The model under review builds one solid part; all positions refer to its coordinate system, in mm. A direction names the side the tool comes from. Round coordinates to 2 decimals unless told otherwise and drop trailing zeros. Order: outer loops, then holes, each group sorted by start corner. A loop starts at its lowest first (then second) coordinate and runs counter-clockwise, first axis right, second up. Notation, with made-up numbers: M -7.75,1 L 43.25,1 A23 ccw 43.25,28 Z; hole C 72,59.5 d3. An arc over 180 degrees is marked long. Answer as CSV lines item,"result". Start each with the question number.
from build123d import *

# Parameters (mm, degrees)
SKETCH_3_W           = 10
SKETCH_3_H           = 35
SKETCH_3_W_2         = 26
SKETCH_3_H_2         = 10
SKETCH_3_W_3         = 38
SKETCH_3_W_4         = 25
EXTRUDE_1_DEPTH      = 1
EXTRUDE_2_DEPTH      = 4
EXTRUDE_2_DEPTH_BACK = 1
SKETCH_5_W           = 25
SKETCH_5_H           = 10
SKETCH_5_W_2         = 10
SKETCH_5_H_2         = 35
EXTRUDE_3_DEPTH      = 2


with BuildPart() as part:
    # 草图3 → 凸台-拉伸1 (new body)
    with BuildSketch(Plane(origin=(0, 0, 0), x_dir=(1, 0, 0), z_dir=(0, 1, 0))):
        with Locations((19, 0)):
            Rectangle(SKETCH_3_W, SKETCH_3_H)
        with Locations((1, 0)):
            Rectangle(SKETCH_3_W_2, SKETCH_3_H_2)
        Polygon((-12, -5), (-12, 5), (-12, 22.5), (-22, 22.5), (-22, 5), (-22, -5), (-22, -22.5), (-12, -22.5), align=None)
        with Locations((-41, 0)):
            Rectangle(SKETCH_3_W_3, SKETCH_3_H_2)
        with Locations((-72.5, 0)):
            Rectangle(SKETCH_3_W_4, SKETCH_3_H_2)
    extrude(amount=EXTRUDE_1_DEPTH)

    # 草图4 → 凸台-拉伸2 (add, two sides)
    with BuildSketch(Plane.XZ) as extrude_2_sk:
        Polygon((13, -18.5), (25, -18.5), (25, 18.5), (13, 18.5), (13, 6), (-11, 6), (-11, 23.5), (-23, 23.5), (-23, 6), (-86, 6), (-86, -6), (-23, -6), (-23, -23.5), (-11, -23.5), (-11, -6), (13, -6), align=None)
        Polygon((14, -17.5), (24, -17.5), (24, 17.5), (14, 17.5), (14, 5), (-12, 5), (-12, 22.5), (-22, 22.5), (-22, 5), (-85, 5), (-85, -5), (-22, -5), (-22, -22.5), (-12, -22.5), (-12, -5), (14, -5), align=None, mode=Mode.SUBTRACT)
    extrude(amount=EXTRUDE_2_DEPTH)
    extrude(extrude_2_sk.sketch, amount=-EXTRUDE_2_DEPTH_BACK)

    # 草图5 → 凸台-拉伸3 (add)
    with BuildSketch(Plane.XZ):
        Polygon((-22, 22.5), (-22, 5), (-20, 5), (-20, -5), (-22, -5), (-22, -22.5), (-12, -22.5), (-12, -5), (-14, -5), (-14, 5), (-12, 5), (-12, 22.5), align=None)
        with Locations((-72.5, 0)):
            Rectangle(SKETCH_5_W, SKETCH_5_H)
        with Locations((19, 0)):
            Rectangle(SKETCH_5_W_2, SKETCH_5_H_2)
    extrude(amount=EXTRUDE_3_DEPTH)


solid = part.part
Item 1: Consider section C-C (x = 0). State the section outline as (y, z) points.
Item 2: Tool access review of faces 1 (the flat face through (13, -2, 12)), 2 (the flat face through (19, -2, 18.5)), 3 (the flat face through (-11, -2, -15)), 4 (the flat face through (-12, -3, -14)): name each direction out of +Z, -Z, +X, -X, +Y, -Y from which nothing blocks a thin tool from reaching the whole face with its end or side.
Item 3: Consider section D-D (z = -0.5). State the section outline as (x, y) points, and give its area (3 significant figures).
Item 4: The part is to be moulded in two halves that separate along Z. For faces 5 (the flat face through (-17, -2, 23.5)), 6 (the flat face through (-11, -2, 15)), 7 (the flat face through (1, -2, -6)), 8 (the flat face through (-17, -2, 0)), say which applies: +Z half, -Z half, draft (parallel to the pull), parting line (faces both ways), or undercut.
Item 5: Consider section B-B (z = 7). State the section outline as (x, y) points, and give its area (3 significant figures).
Item 6: For pin 1 (5 mm diameter, centred on x = -18.5, z = 4, fed in from -Y); pin 2 (6 mm diameter, centred on x = 4, z = 4, fed in from -Y); pin 3 (3 mm diameter, centred on x = -48, z = 0.5, fed in from -Y); pin 4 (3 mm diameter, centred on x = -52.5, y = -2, fed in from -Z), all flat-tipped, find the tip position at first contact; note any pin that passes through.
Item 7: Wall thickness on probe 1 along X at (y, z) = (-0.6, -3.5); probe 2 along X at (y, z) = (-2.3, 12.5); probe 3 along Z at (x, y) = (7, -0.2): over which ranges is each line inside the solid? List them lowest first. Write a range as [from, to].
Reported:
1,outline,"M -4,-6 L 1,-6 L 1,6 L -4,6 L -4,5 L 0,5 L 0,-5 L -4,-5 Z"
2,face 1,"+Z, +Y, -Y"
2,face 2,"+Z, +X, +Y, -Y"
2,face 3,"-Z, +Y, -Y"
2,face 4,"-Y"
3,outline,"M -86,-4 L -85,-4 L -85,-2 L -60,-2 L -60,0 L -20,0 L -20,-2 L -14,-2 L -14,0 L 14,0 L 14,-2 L 24,-2 L 24,-4 L 25,-4 L 25,1 L -86,1 Z"
3,area,"201 mm²"
4,face 5,"+Z half"
4,face 6,"draft"
4,face 7,"-Z half"
4,face 8,"undercut"
5,outline,"M -23,-4 L -22,-4 L -22,-2 L -12,-2 L -12,-4 L -11,-4 L -11,1 L -23,1 Z; M 13,-4 L 14,-4 L 14,-2 L 24,-2 L 24,-4 L 25,-4 L 25,1 L 13,1 Z"
5,area,"80.0 mm²"
6,pin 1,"stops at y = -2"
6,pin 2,"stops at y = -4"
6,pin 3,"stops at y = 0"
6,pin 4,"stops at z = -6"
7,probe 1,"x = [-86, -60], [-20, -14], [14, 25]"
7,probe 2,"x = [-23, -22], [-12, -11], [13, 14], [24, 25]"
7,probe 3,"z = [-6, -5], [5, 6]"
